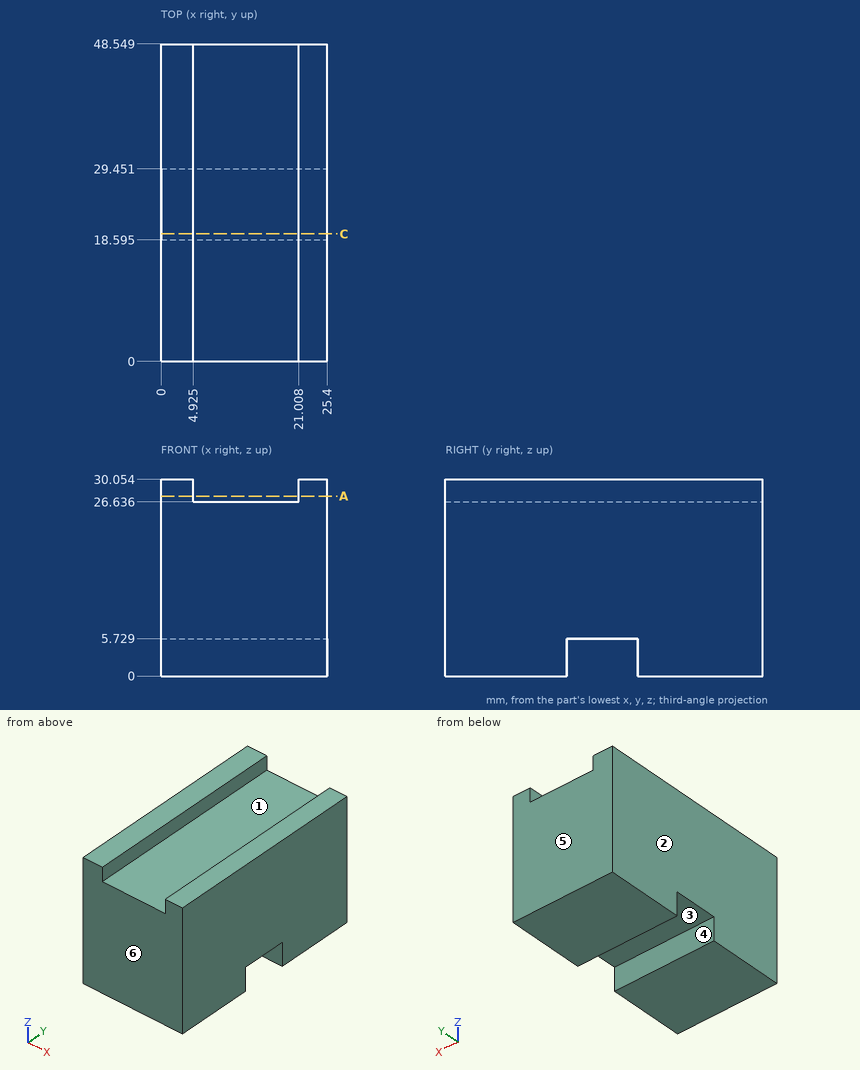
Design review of the part shown in the three views and the two pictorial views. Dimensions are in mm from the part's minimum x, y and z. A direction names the side the tool comes from. Give positions to 0.01 mm unless a question says otherwise; leave off trailing zeros. Write each loop counter-clockwise with the first axis right and the second up, starting at its lowest first coordinate (ties: lowest second). Pieces come first, ordered by that corner, then holes. Notation, with made-up numbers: M 25.5,6 L 49.5,6 A11 ccw 49.5,16 Z; hole C 26.25,24 d4. An arc over 180 degrees is marked long. Return JSON: item names as keys, results as strings. Group by question number.
Item 1: Clearance check with a flat-ended pin moving along its axis: pin 1 Ø8 at (x, y) = (13.5, 22) entering from +Z. State where the tip first meets the part, or that it passes through.
Item 2: Wall thickness on line 1 along X through (y, z) = (8, 29) (1 decimal); line 2 along Z through (x, y) = (15, 29); line 3 along Z through (x, y) = (16.25, 7.5): over which ranges is each line inside the solid? List them lowest first.
Item 3: Tool access review of the marked faces 1 and 2: name each direction out of +Z, -Z, +X, -X, +Y, -Y from which nothing blocks a thin tool from reaching the whole face with its end or side.
Item 4: Take a section at A-A (z = 27.5). Give the boundary of the cut face in (x, y) (1 decimal).
Item 5: The part is to be moulded in two halves that separate along Y. For the marked faces 3, 4, 5 and 6, say which applies: pulls with the +Y half, pulls with the -Y half, needs draft (parallel to the pull), parting line crosses it, or undercut.
Item 6: Take a section at C-C (y = 19.5). Give the boundary of the cut face in (x, z) (1 decimal), plus the area to 3 significant figures.
Return value:
{
 "1": {"pin 1": "stops at z = 26.64"},
 "2": {"line 1": "x = 0 to 4.9, 21 to 25.4", "line 2": "z = 5.73 to 26.64", "line 3": "z = 0 to 26.64"},
 "3": {"face 1": "+Z, +Y, -Y", "face 2": "+Z, -Z, -X, +Y, -Y"},
 "4": {"outline": "M 0,0 L 4.9,0 L 4.9,48.5 L 0,48.5 Z; M 21,0 L 25.4,0 L 25.4,48.5 L 21,48.5 Z"},
 "5": {"face 3": "undercut", "face 4": "undercut", "face 5": "pulls with the +Y half", "face 6": "pulls with the -Y half"},
 "6": {"outline": "M 0,5.7 L 25.4,5.7 L 25.4,30.1 L 21,30.1 L 21,26.6 L 4.9,26.6 L 4.9,30.1 L 0,30.1 Z", "area": "563 mm2"}
}
